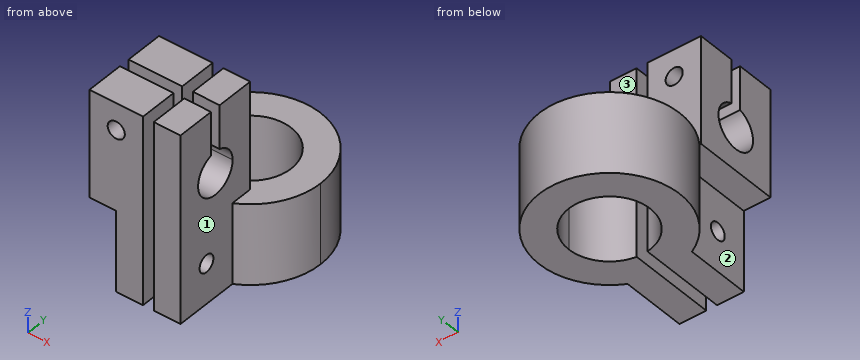
```python
from build123d import *

# Parameters (mm, degrees)
F1_DEPTH  = 15
F2_R      = 1.6
F3_DEPTH  = 20
F4_W      = 5
F4_H      = 16.1112473921
F5_DEPTH  = 20
F6_W      = 16.1112473921
F6_H      = 20
F7_DEPTH  = 5
F9_DEPTH  = 20
F10_R     = 1.6
F11_DEPTH = 20


with BuildPart() as f1:
    # F0 (on Top) → F1 (new body)
    with BuildSketch(Plane.XY):
        with BuildLine():
            Line((-1, -23.6451706729), (-1, -13.0617762957))
            ThreePointArc((-1, -13.0617762957), (-3.570951256, -12.6039004728), (-6, -11.6451706729))
            Line((-6, -11.6451706729), (-6, -23.6451706729))
            Line((-6, -23.6451706729), (-1, -23.6451706729))
        make_face()
        with BuildLine():
            ThreePointArc((6, -11.6451706729), (3.570951256, -12.6039004728), (1, -13.0617762957))
            Line((1, -13.0617762957), (1, -23.6451706729))
            Line((1, -23.6451706729), (6, -23.6451706729))
            Line((6, -23.6451706729), (6, -11.6451706729))
        make_face()
        with BuildLine():
            ThreePointArc((-1, -7.5339232807), (-5.0079936102, 5.7166423712), (7.6, 0))
            ThreePointArc((7.6, 0), (5.7166423712, -5.0079936102), (1, -7.5339232807))
            Line((1, -7.5339232807), (1, -13.0617762957))
            ThreePointArc((1, -13.0617762957), (3.570951256, -12.6039004728), (6, -11.6451706729))
            ThreePointArc((6, -11.6451706729), (11.1850346446, -6.8194574564), (13.1, 0))
            ThreePointArc((13.1, 0), (-6.8194574564, 11.1850346446), (-6, -11.6451706729))
            ThreePointArc((-6, -11.6451706729), (-3.570951256, -12.6039004728), (-1, -13.0617762957))
            Line((-1, -13.0617762957), (-1, -7.5339232807))
        make_face()
    extrude(amount=F1_DEPTH)

    # F2 (on face) → F3 (cut)
    with BuildSketch(Plane.YZ.offset(6)):
        with Locations((-17.6451706729, 7.5)):
            Circle(F2_R)
    extrude(amount=-F3_DEPTH, mode=Mode.SUBTRACT)

    # F4 (on face) → F5 (join)
    with BuildSketch(Plane.XY.offset(15)):
        with Locations((3.5, -15.5895469768)):
            Rectangle(F4_W, F4_H)
        with Locations((-3.5, -15.5895469768)):
            Rectangle(F4_W, F4_H)
    extrude(amount=F5_DEPTH)

    # F6 (on face) → F7 (join)
    with BuildSketch(Plane(origin=(-6, 0, 0), x_dir=(0, -1, 0), z_dir=(-1, 0, 0))):
        with Locations((15.5895469768, 25)):
            Rectangle(F6_W, F6_H)
    extrude(amount=F7_DEPTH)

    # F8 (on face) → F9 (cut)
    with BuildSketch(Plane.YZ.offset(6)):
        with BuildLine():
            ThreePointArc((-16.5895469768, 26.8729833462), (-18.0390367196, 19.8377223398), (-11.5895469768, 23))
            ThreePointArc((-11.5895469768, 23), (-12.4272693166, 25.4494897428), (-14.5895469768, 26.8729833462))
            Line((-14.5895469768, 26.8729833462), (-16.5895469768, 26.8729833462))
        make_face()
        with BuildLine():
            Line((-16.5895469768, 26.8729833462), (-14.5895469768, 26.8729833462))
            ThreePointArc((-14.5895469768, 26.8729833462), (-15.5895469768, 27), (-16.5895469768, 26.8729833462))
        make_face()
        with BuildLine():
            ThreePointArc((-16.5895469768, 26.8729833462), (-15.5895469768, 27), (-14.5895469768, 26.8729833462))
            Line((-14.5895469768, 26.8729833462), (-14.5895469768, 35))
            Line((-14.5895469768, 35), (-16.5895469768, 35))
            Line((-16.5895469768, 35), (-16.5895469768, 26.8729833462))
        make_face()
    extrude(amount=-F9_DEPTH, mode=Mode.SUBTRACT)

    # F10 (on face) → F11 (cut)
    with BuildSketch(Plane.XZ.offset(23.6451706729)):
        with Locations((-6, 30)):
            Circle(F10_R)
    extrude(amount=-F11_DEPTH, mode=Mode.SUBTRACT)


solid = f1.part
```
Geometry check sheet. Reference: the model listing, model coordinates, mm. Face numbers are marked on the shaded views. A direction names the side the tool comes from. Give positions to 0.01 mm unless a question says otherwise; leave off trailing zeros. Write each loop counter-clockwise with the first axis right and the second up, starting at its lowest first coordinate (ties: lowest second). Pieces come first, ordered by that corner, then holes. Notation, with made-up numbers: (-20, 40.25) -> (-8, 40.25) arc R23 ccw to (-8, 54.25) -> close; hole circle Ø5 at (-2, 66). An arc over 180 degrees is marked (long way). One line per question, with ' | ' between items.
Item 1: Sectioned sample at D-D, the plane x = -7. Record the boundary of the cut face in (y, z), plus the area to 3 significant figures.
Determined:
outline: (-23.65, 15) -> (-11.07, 15) -> (-11.07, 0) -> (-2.96, 0) -> (-2.96, 15) -> (-7.53, 15) -> (-7.53, 28.75) -> (-14.59, 28.75) -> (-14.59, 26.87) arc R4 cw (long way) to (-16.59, 26.87) -> (-16.59, 28.75) -> (-23.65, 28.75) -> close; (-23.65, 31.25) -> (-16.59, 31.25) -> (-16.59, 35) -> (-23.65, 35) -> close; (-14.59, 31.25) -> (-7.53, 31.25) -> (-7.53, 35) -> (-14.59, 35) -> close; (2.96, 0) -> (11.07, 0) -> (11.07, 15) -> (2.96, 15) -> close | area: 464 mm^2
Item 2: Sectioned sample at A-A, the plane z = 30. Record the boundary of the cut face in (x, y).
Determined:
outline: (-11, -23.65) -> (-7.6, -23.65) -> (-7.6, -16.59) -> (-11, -16.59) -> close; (-11, -14.59) -> (-7.6, -14.59) -> (-7.6, -7.53) -> (-11, -7.53) -> close; (-4.4, -23.65) -> (-1, -23.65) -> (-1, -16.59) -> (-4.4, -16.59) -> close; (-4.4, -14.59) -> (-1, -14.59) -> (-1, -7.53) -> (-4.4, -7.53) -> close; (1, -23.65) -> (6, -23.65) -> (6, -16.59) -> (1, -16.59) -> close; (1, -14.59) -> (6, -14.59) -> (6, -7.53) -> (1, -7.53) -> close
Item 3: Access from +Z, -Z, +X, -X, +Y, -Y to the whole of each face (thin tool, end or side, straight path). Record for the marked faces 1, 2 and 3.
Determined:
face 1: +Z, +X, -Y | face 2: -Z, -X, -Y | face 3: +Z, +X, -X, +Y
Item 4: Scan lines: line 1 along Y through (x, z) = (4.75, 23); line 2 along X through (y, z) = (-18, 4); line 3 along X through (y, z) = (-19.5, 31). Record each from-to range of solid material in increasing order.
Determined:
line 1: -23.65 to -19.59, -11.59 to -7.53 | line 2: -6 to -1, 1 to 6 | line 3: -11 to -7.25, -4.75 to -1, 1 to 6
Item 5: Depth check by flat-ended pin: pin 1 (8 mm diameter, centred on x = -6.5, z = 24.5, fed in from +Y); pin 2 (6 mm diameter, centred on x = 10.5, z = 30, fed in from +Y); pin 3 (5 mm diameter, centred on y = -12.5, z = 29, fed in from -X); pin 4 (4 mm diameter, centred on x = -8, y = -12, fed in from -Z). Enter the tip coordinate at first touch or a pass-through.
Determined:
pin 1: y = -7.53 | pin 2: through | pin 3: x = -11 | pin 4: z = 0
Item 6: Sectioned sample at C-C, the plane y = 1. Record the boundary of the cut face in (x, z), plus the area to 3 significant figures.
Determined:
outline: (-13.06, 0) -> (-7.53, 0) -> (-7.53, 15) -> (-13.06, 15) -> close; (7.53, 0) -> (13.06, 0) -> (13.06, 15) -> (7.53, 15) -> close | area: 166 mm^2
Item 7: Sectioned sample at B-B, the plane x = 4.5. Record the boundary of the cut face in (y, z).
Determined:
outline: (-23.65, 0) -> (-6.12, 0) -> (-6.12, 15) -> (-7.53, 15) -> (-7.53, 35) -> (-14.59, 35) -> (-14.59, 26.87) arc R4 cw (long way) to (-16.59, 26.87) -> (-16.59, 35) -> (-23.65, 35) -> close; (6.12, 0) -> (12.3, 0) -> (12.3, 15) -> (6.12, 15) -> close; hole circle Ø3.2 at (-17.65, 7.5)
